Check sheet for the modelled part. Datum: model origin and axes. Units: mm. A direction names the side the tool comes from. Give positions to 0.01 mm unless a question says otherwise; leave off trailing zeros. Order: outer loops, then holes, each group sorted by start corner. A loop starts at its lowest first (then second) coordinate and runs counter-clockwise, first axis right, second up.
```python
from build123d import *

# Parameters (mm, degrees)
F0_W      = 50.8
F0_H      = 50.8
F1_DEPTH  = 50.8
F2_R      = 10.8954734827
F3_DEPTH  = 25.4
F4_W      = 25.4
F4_H      = 25.4
F5_DEPTH  = 25.4
F6_DEPTH  = 12.7
F7_DEPTH  = 38.1
F8_W      = 26.3517424464
F8_H      = 21.1959667504
F9_DEPTH  = 12.7
F10_R     = 11.2387805826
F11_DEPTH = 12.7


with BuildPart() as f1:
    # F0 (on Front) → F1 (new body)
    with BuildSketch(Plane.XZ):
        with Locations((-25.4, 25.4)):
            Rectangle(F0_W, F0_H)
    extrude(amount=F1_DEPTH)

    # F2 (on face) → F3 (cut)
    with BuildSketch(Plane.XY.offset(50.8)):
        with Locations((-25.4, -25.4)):
            Circle(F2_R)
    extrude(amount=-F3_DEPTH, mode=Mode.SUBTRACT)

    # F4 (on face) → F5 (join)
    with BuildSketch(Plane.XZ.offset(50.8)):
        with Locations((-25.4, 25.4)):
            Rectangle(F4_W, F4_H)
    extrude(amount=F5_DEPTH)

    # F6 (add): a face of the model
    f6_faces = [f1.faces().sort_by_distance(p)[0] for p in [
        (-25.4, -76.2, 25.4),
    ]]
    extrude(f6_faces, amount=F6_DEPTH)

    # F7 (cut): a face of the model
    f7_faces = [f1.faces().sort_by_distance(p)[0] for p in [
        (-25.4, -88.9, 25.4),
    ]]
    extrude(f7_faces, amount=-F7_DEPTH, mode=Mode.SUBTRACT)

    # F8 (on face) → F9 (join)
    with BuildSketch(Plane.XZ.offset(50.8)):
        with Locations((-25.3969691694, 25.1105371863)):
            Rectangle(F8_W, F8_H)
    extrude(amount=F9_DEPTH)

    # F10 (on face) → F11 (join)
    with BuildSketch(Plane.YZ):
        with Locations((-25.5879238248, 23.8693319261)):
            Circle(F10_R)
    extrude(amount=F11_DEPTH)


solid = f1.part
```
Q1. Go/stop test with flat-tipped pins: P1, Ø10, axis at x = -31, y = -56, coming from the +Z side; P2, Ø6.5, axis at x = -30.5, y = -30, coming from the +Z side; P3, Ø4, axis at x = -28, y = -58.5, coming from the -Z side. Record where each tip stops, or that it passes through.
Q2. Sectioned sample at B-B, the plane x = -13.5. Record the cut outline in (y, z).
Q3. Tool access check on faces 1 (the flat face through (-26, -25, 25.4)), 2 (the cylindrical face through (6.261, -33.871, 31.465)), 3 (the flat face through (-26, -57, 35.709)), 4 (the flat face through (-38.573, -57, 25)). Record the directions out of +Z, -Z, +X, -X, +Y, -Y that give a thin tool (end or side, any length) a straight path to the whole face; none if there is none.
Q4. Draft check along X on faces 5 (the flat face through (-14, -25, 50.8)), 6 (the cylindrical face through (-19.543, -16.213, 38.278)), 7 (the flat face through (0, -25, 36)). Enter one of: pulls with the +X half, pulls with the -X half, needs draft (parallel to the pull), parting line crosses it, or undercut.
Q5. Sectioned sample at A-A, the plane z = 31.5. Record the cut outline in (x, y).
Q6. Material ranges on line 1 (X direction, y = -25, z = 31); line 2 (Y direction, x = -25.4, z = 45.75); line 3 (X direction, y = -25, z = 45), recorded low to high.
Q7. Sectioned sample at D-D, the plane z = 7.5. Record the cut outline in (x, y).
Q8. Sectioned sample at C-C, the plane y = -30. Record the cut outline in (x, z).
Filled in:
1. P1: stops at z = 35.71
1. P2: stops at z = 25.4
1. P3: stops at z = 14.51
2. outline: (-63.5, 14.51) - (-50.8, 14.51) - (-50.8, 0) - (0, 0) - (0, 50.8) - (-50.8, 50.8) - (-50.8, 35.71) - (-63.5, 35.71) - close
3. face 1: +Z
3. face 2: +X
3. face 3: +Z, +X, -X, -Y
3. face 4: +Z, -Z, -X, -Y
4. face 5: needs draft
4. face 6: undercut
4. face 7: pulls with the +X half
5. outline: (-50.8, -50.8) - (-38.57, -50.8) - (-38.57, -63.5) - (-12.22, -63.5) - (-12.22, -50.8) - (0, -50.8) - (0, -33.84) - (12.7, -33.84) - (12.7, -17.34) - (0, -17.34) - (0, 0) - (-50.8, 0) - close; hole circle Ø21.79 at (-25.4, -25.4)
6. line 1: x = -50.8 to -36.29, -14.51 to 12.7
6. line 2: y = -50.8 to -36.3, -14.5 to 0
6. line 3: x = -50.8 to -36.29, -14.51 to 0
7. outline: (-50.8, -50.8) - (0, -50.8) - (0, 0) - (-50.8, 0) - close
8. outline: (-50.8, 0) - (0, 0) - (0, 13.53) - (12.7, 13.53) - (12.7, 34.21) - (0, 34.21) - (0, 50.8) - (-15.52, 50.8) - (-15.52, 25.4) - (-35.28, 25.4) - (-35.28, 50.8) - (-50.8, 50.8) - close
